```python
from build123d import *

# Parameters (mm, degrees)
SKETCH1_W           = 100
SKETCH1_H           = 70
BOSS_EXTRUDE1_DEPTH = 5
FILLET1_R           = 4
SKETCH3_W           = 20
SKETCH3_H           = 27
CUT_EXTRUDE1_DEPTH  = 5
CUT_EXTRUDE2_DEPTH  = 96
SKETCH6_W           = 70
SKETCH6_H           = 3
CUT_EXTRUDE3_DEPTH  = 4


with BuildPart() as part:
    # Sketch1 → Boss-Extrude1 (new body)
    with BuildSketch(Plane(origin=(0, 0, 0), x_dir=(0, 1, 0), z_dir=(0, 0, 1))):
        Rectangle(SKETCH1_W, SKETCH1_H)
    extrude(amount=BOSS_EXTRUDE1_DEPTH)

    # Fillet1
    fillet1_edges = [part.edges().sort_by_distance(p)[0] for p in [
        (35, 50, 2.5),
        (35, -50, 2.5),
        (-35, -50, 2.5),
        (-35, 50, 2.5),
    ]]
    fillet(fillet1_edges, radius=FILLET1_R)

    # Sketch3 → Cut-Extrude1 (cut)
    with BuildSketch(Plane(origin=(0, 0, 0), x_dir=(1, 0, 0), z_dir=(0, 0, -1))):
        with Locations((1.3, 7.45)):
            Rectangle(SKETCH3_W, SKETCH3_H)
    extrude(amount=-CUT_EXTRUDE1_DEPTH, mode=Mode.SUBTRACT)

    # Sketch5 → Cut-Extrude2 (cut)
    with BuildSketch(Plane(origin=(0, 50, 0), x_dir=(-1, 0, 0), z_dir=(0, 1, 0))):
        Polygon((-35, 3), (-33, 3), (-33, 2), (-34, 2), (-34, 1), (-33, 1), (-33, 0), (-35, 0), align=None)
        Polygon((35, 3), (35, 0), (33, 0), (33, 1), (34, 1), (34, 2), (33, 2), (33, 3), align=None)
    extrude(amount=-CUT_EXTRUDE2_DEPTH, mode=Mode.SUBTRACT)

    # Sketch6 → Cut-Extrude3 (cut)
    with BuildSketch(Plane(origin=(0, 50, 0), x_dir=(-1, 0, 0), z_dir=(0, 1, 0))):
        with Locations((0, 1.5)):
            Rectangle(SKETCH6_W, SKETCH6_H)
    extrude(amount=-CUT_EXTRUDE3_DEPTH, mode=Mode.SUBTRACT)


solid = part.part
```
Geometry check sheet. Reference: the model listing, model coordinates, mm. A direction names the side the tool comes from. Coordinates: 2 decimals unless noted, no trailing zeros. Order: outer loops, then holes, each group sorted by start corner. A loop starts at its lowest first (then second) coordinate and runs counter-clockwise, first axis right, second up. Notation, with made-up numbers: (80.25, -27) - (89.25, -27) arc R16 ccw to (89.25, 0) - close; hole circle Ø2 at (38, 68.5). An arc over 180 degrees is marked (long way). Answer in a Markdown table with one row per item. Add a question column.
1. Material ranges on L1, parallel to X at y = 5.5, z = 2.6; L2, parallel to Y at x = 4.5, z = 0.4; L3, parallel to Y at x = 5, z = 4.5, recorded low to high. Write a range as [from, to].
2. Gauge pin test, flat ends, axial feed: pin 1 Ø0.5 at (y, z) = (7, 1.5) entering from +X; pin 2 Ø1.5 at (x, z) = (23, 2) entering from +Y; pin 3 Ø0.8 at (y, z) = (-9, 0.5) entering from -X; pin 4 Ø2.5 at (x, z) = (14, 2) entering from +Y. Record the tip position at first contact, or that the pin passes through.
3. Section check B-B (y = -12). Enter the section's corners in (x, z), plus the area to 3 significant figures.
4. Section check D-D (y = 14). Enter the section's corners in (x, z).
5. Section check A-A (x = 1.5). Enter the section's corners in (y, z).
6. Access from +Z, -Z, +X, -X, +Y, -Y to the whole of each face (thin tool, end or side, straight path). Record for faces 5 (the face through (0, -50, 2)), 6 (the face through (11.3, -7, 2)), 7 (the face through (0, 46, 2)), 8 (the face through (35, -1, 4)), 9 (the face through (0, 48, 3)).
7. Section check C-C (z = 4.2). Enter the section's corners in (x, y).
8. Draft check along Z on faces 1 (the face through (0, 10, 5)), 2 (the face through (-34.2, -46, 1.5)), 3 (the face through (34.2, -46, 1.5)), 4 (the face through (0, 8, 0)). Enter one of: +Z half, -Z half, draft (parallel to the pull), parting line (faces both ways), or undercut.
Data:
| question | item | result |
|---|---|---|
| 1 | L1 | x = [-33, -8.7], [11.3, 33] |
| 1 | L2 | y = [-50, -20.95], [6.05, 46] |
| 1 | L3 | y = [-50, -20.95], [6.05, 50] |
| 2 | pin 1 | stops at x = 34 |
| 2 | pin 2 | stops at y = 46 |
| 2 | pin 3 | stops at x = -33 |
| 2 | pin 4 | stops at y = 50 |
| 3 | outline | (-35, 3) - (-33, 3) - (-33, 2) - (-34, 2) - (-34, 1) - (-33, 1) - (-33, 0) - (-8.7, 0) - (-8.7, 5) - (-35, 5) - close; (11.3, 0) - (33, 0) - (33, 1) - (34, 1) - (34, 2) - (33, 2) - (33, 3) - (35, 3) - (35, 5) - (11.3, 5) - close |
| 3 | area | 240 mm² |
| 4 | outline | (-35, 3) - (-33, 3) - (-33, 2) - (-34, 2) - (-34, 1) - (-33, 1) - (-33, 0) - (33, 0) - (33, 1) - (34, 1) - (34, 2) - (33, 2) - (33, 3) - (35, 3) - (35, 5) - (-35, 5) - close |
| 5 | outline | (-50, 0) - (-20.95, 0) - (-20.95, 5) - (-50, 5) - close; (6.05, 0) - (46, 0) - (46, 3) - (50, 3) - (50, 5) - (6.05, 5) - close |
| 6 | face 5 | +Z, -Z, +X, -X, -Y |
| 6 | face 6 | +Z, -Z |
| 6 | face 7 | -Z, +X, -X, +Y |
| 6 | face 8 | +Z, -Z, +X, +Y, -Y |
| 6 | face 9 | +Y |
| 7 | outline | (-35, -46) arc R4 ccw to (-31, -50) - (31, -50) arc R4 ccw to (35, -46) - (35, 46) arc R4 ccw to (31, 50) - (-31, 50) arc R4 ccw to (-35, 46) - close; hole (-8.7, -20.95) - (11.3, -20.95) - (11.3, 6.05) - (-8.7, 6.05) - close |
| 8 | face 1 | +Z half |
| 8 | face 2 | undercut |
| 8 | face 3 | undercut |
| 8 | face 4 | -Z half |
